Input: part model. Units: mm. Frame: model coordinates. Face numbers are marked on the shaded views. Round coordinates to 2 decimals unless told otherwise and drop trailing zeros. Loops run counter-clockwise (first coordinate to the right, second up) from the corner with the lowest first, then second, coordinate; pieces in that order, holes last.
1) Section C-C, the plane y = -183. Return loops of the section in (x, z), and give its area (3 significant figures).
2) Section B-B, the plane z = 53.5. Return loops of the section in (x, y), and give its area (3 significant figures).
3) Draft query along X for the marked faces 1, 2 and 3. Return one class per face: pulls with the +X half, pulls with the -X half, needs draft (parallel to the pull), parting line crosses it, or undercut.
4) Section A-A, the plane z = -50. Return loops of the section in (x, y).
5) Ray query, line 1 along X through (y, z) = (-267.5, 37); line 2 along Y through (x, z) = (-78.5, 49); line 3 along Z through (x, y) = (-57, -172). Return the intervals inside material, ascending.
6) Section D-D, the plane x = -38.5. Return loops of the section in (y, z).
7) First-contact query: pin 1 (0.8 mm diameter, centred on x = -146.5, z = -62, fed in from -Y); pin 2 (0.8 mm diameter, centred on x = 147, z = -62.5, fed in from +Y); pin 3 (12 mm diameter, centred on x = 107, z = -7.5, fed in from -Y). Flat tips, straight axial feed; report the tip coordinate or a pass-through.
from build123d import *

# Parameters (mm, degrees)
F2_DEPTH      = 215.9
F3_DEPTH      = 76.2
F5_DEPTH      = 375.92
F5_DEPTH_BACK = 25.4
F6_W          = 2.794
F6_H          = 88.9
F7_DEPTH      = 348.996
F8_W          = 32.20243752
F8_H          = 2.794
F9_DEPTH      = 348.996
F10_W         = 254
F10_H         = 32.20243752
F11_DEPTH     = 25.4
F12_R         = 3.175
F13_DEPTH     = 25.4
F15_DEPTH     = 25.4
F16_R         = 6.35
F17_DEPTH     = 25.4


with BuildPart() as f2:
    # F1 (on Front) → F2 (new body, symmetric)
    with BuildSketch(Plane.XZ):
        Polygon((177.8, 63.5), (-177.8, 63.5), (-177.8, -63.5), (-174.498, -63.5), (-174.498, 60.198), (174.498, 60.198), (174.498, -63.5), (177.8, -63.5), align=None)
    extrude(amount=F2_DEPTH, both=True)

    # F3 (add): a face of the model
    f3_faces = [f2.faces().sort_by_distance(p)[0] for p in [
        (176.149, -215.9, -59.7240185382),
    ]]
    extrude(f3_faces, amount=F3_DEPTH)

    # F4 (on face) → F5 (cut, two sides)
    with BuildSketch(Plane.YZ.offset(177.8)) as f5_sk:
        Polygon((-292.1, -63.5), (-215.9, -63.5), (-292.1, 63.5), align=None)
    extrude(amount=-F5_DEPTH, mode=Mode.SUBTRACT)
    extrude(f5_sk.sketch, amount=F5_DEPTH_BACK, mode=Mode.SUBTRACT)

    # F6 (on face) → F7 (join, through all)
    with BuildSketch(Plane.YZ.offset(-174.498)):
        with Locations((214.503, 15.748)):
            Rectangle(F6_W, F6_H)
    extrude(amount=F7_DEPTH)

    # F8 (on face) → F9 (join, through all)
    with BuildSketch(Plane(origin=(174.498, 0, 0), x_dir=(0, -1, 0), z_dir=(-1, 0, 0))):
        with Locations((0, -62.103)):
            Rectangle(F8_W, F8_H)
    extrude(amount=F9_DEPTH)

    # F10 (on face) → F11 (cut)
    with BuildSketch(Plane(origin=(0, 0, -63.5), x_dir=(1, 0, 0), z_dir=(0, 0, -1))):
        Rectangle(F10_W, F10_H)
    extrude(amount=-F11_DEPTH, mode=Mode.SUBTRACT)

    # F12 (on face) → F13 (cut)
    with BuildSketch(Plane(origin=(0, 0, -63.5), x_dir=(1, 0, 0), z_dir=(0, 0, -1))):
        with Locations((149.098, 0)):
            Circle(F12_R)
    extrude(amount=-F13_DEPTH, mode=Mode.SUBTRACT)

    # F14 (on face) → F15 (cut)
    with BuildSketch(Plane(origin=(0, 0, -63.5), x_dir=(1, 0, 0), z_dir=(0, 0, -1))):
        with BuildLine():
            ThreePointArc((-152.273, 0), (-149.098, -3.175), (-145.923, 0))
            ThreePointArc((-145.923, 0), (-149.098, 3.175), (-152.273, 0))
        make_face()
    extrude(amount=-F15_DEPTH, mode=Mode.SUBTRACT)

    # F16 (on face) → F17 (cut)
    with BuildSketch(Plane(origin=(0, 0, 60.198), x_dir=(1, 0, 0), z_dir=(0, 0, -1))):
        with Locations((149.098, 0)):
            Circle(F16_R)
        with Locations((-149.098, 0)):
            Circle(F16_R)
    extrude(amount=-F17_DEPTH, mode=Mode.SUBTRACT)


solid = f2.part
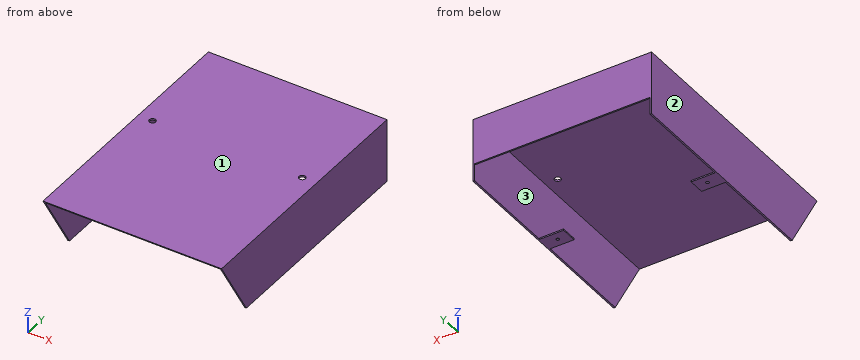
Final values:
1. outline: (-177.8, -63.5) - (-174.5, -63.5) - (-174.5, 60.2) - (174.5, 60.2) - (174.5, -63.5) - (177.8, -63.5) - (177.8, 63.5) - (-177.8, 63.5) - close
1. area: 1,990 mm2
2. outline: (-177.8, -286.1) - (-174.5, -286.1) - (-174.5, 213.11) - (174.5, 213.11) - (174.5, -286.1) - (177.8, -286.1) - (177.8, 215.9) - (-177.8, 215.9) - close
2. area: 4,290 mm2
3. face 1: needs draft
3. face 2: pulls with the -X half
3. face 3: undercut
4. outline: (-177.8, -224) - (-174.5, -224) - (-174.5, 215.9) - (-177.8, 215.9) - close; (174.5, -224) - (177.8, -224) - (177.8, 215.9) - (174.5, 215.9) - close
5. line 1: x = -177.8 to -174.5, 174.5 to 177.8
5. line 2: y = 213.11 to 215.9
5. line 3: z = 60.2 to 63.5
6. outline: (-292.1, 63.5) - (-290.12, 60.2) - (213.11, 60.2) - (213.11, -28.7) - (215.9, -28.7) - (215.9, 63.5) - close
7. pin 1: stops at y = -16.1
7. pin 2: stops at y = 16.1
7. pin 3: stops at y = 213.11
